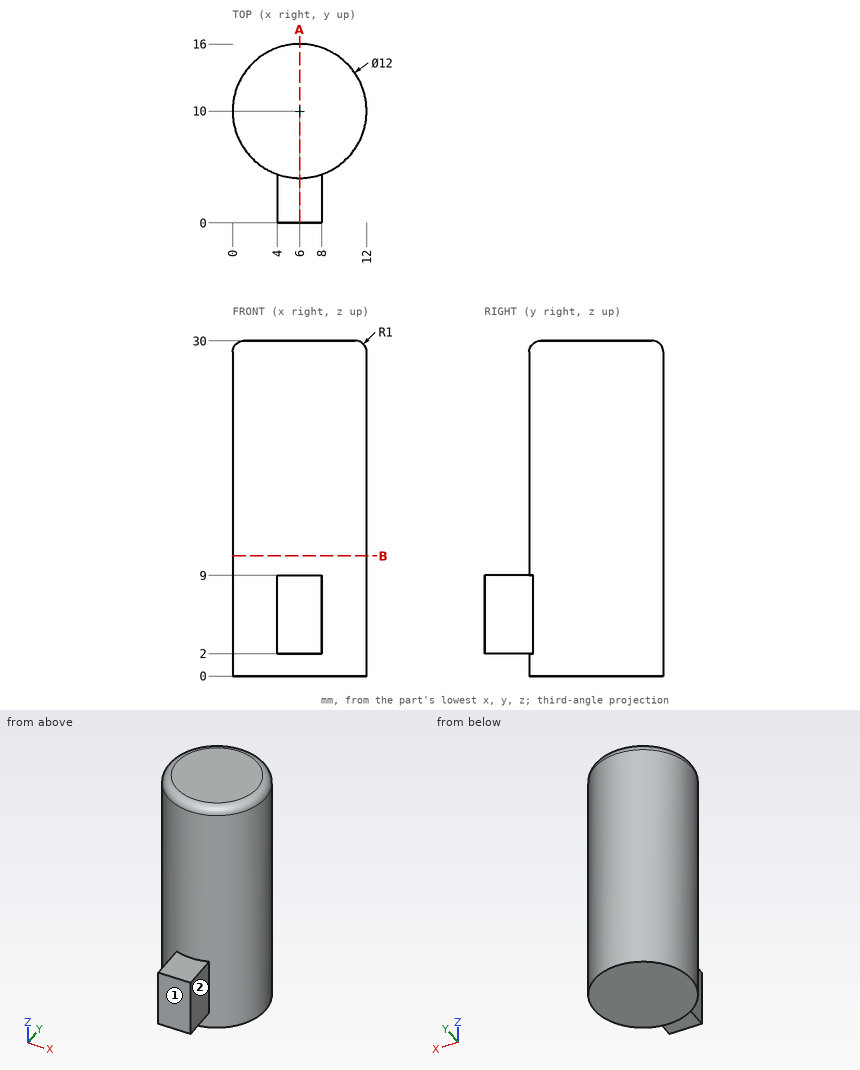
Input: dimensioned drawing with shaded views. Units: mm. Origin: part minimum x, y, z. A direction names the side the tool comes from. Give positions to 0.01 mm unless a question says otherwise; leave off trailing zeros. Write each loop counter-clockwise with the first axis right and the second up, starting at its lowest first coordinate (ties: lowest second). Pieces come first, ordered by that corner, then holes. Notation, with made-up numbers: M 84,-14.5 L 93,-14.5 A27 cw 93,9.5 Z; hole C 21.5,-38 d11. An arc over 180 degrees is marked long. Return JSON: item names as keys, results as strings. Group by question number.
1) Set-up query: the marked faces 1 and 2. Return all of +Z, -Z, +X, -X, +Y, -Y with unobstructed straight access to the full face (end or side cutting, diameter ignored); none if empty.
2) Material intervals for line 1 along X through (y, z) = (2, 4); line 2 along Y through (x, z) = (6, 19.5); line 3 along X through (y, z) = (11.75, 25.5), sorted ascending. Write a range as [from, to].
3) Cut plane A-A, the plane x = 6. Output: boundary loops of the cut face in (y, z), plus the area to 3 significant figures.
4) Cut plane B-B, the plane z = 10.75. Output: boundary loops of the cut face in (x, y).
5) Pin query (flat end, axial travel): P1, Ø4, axis at x = 3.5, y = 3.5, coming from the -Z side; P2, Ø8, axis at y = 5, z = 25, coming from the -X side; P3, Ø5, axis at y = 3, z = 4.5, coming from the -X side; P4, Ø3, axis at x = 3, z = 23.5, coming from the -Y side. Return the tip coordinate at first contact, or that it passes through.
Recorded:
{
 "1": {"face 1": "+Z, -Z, +X, -X, -Y", "face 2": "+Z, -Z, +X, -Y"},
 "2": {"line 1": "x = [4, 8]", "line 2": "y = [4, 16]", "line 3": "x = [0.26, 11.74]"},
 "3": {"outline": "M 0,2 L 4,2 L 4,0 L 16,0 L 16,29 A1 ccw 15,30 L 5,30 A1 ccw 4,29 L 4,9 L 0,9 Z", "area": "388 mm²"},
 "4": {"outline": "C 6,10 d12"},
 "5": {"P1": "stops at z = 0", "P2": "stops at x = 0.08", "P3": "stops at x = 2.03", "P4": "stops at y = 4.19"}
}
